For this review, take the finished solid that the model builds, in its own axes (mm). Face numbers are marked on the shaded views. A direction names the side the tool comes from. Give positions to 0.01 mm unless a question says otherwise; leave off trailing zeros. Order: outer loops, then holes, each group sorted by start corner. A loop starts at its lowest first (then second) coordinate and runs counter-clockwise, first axis right, second up.
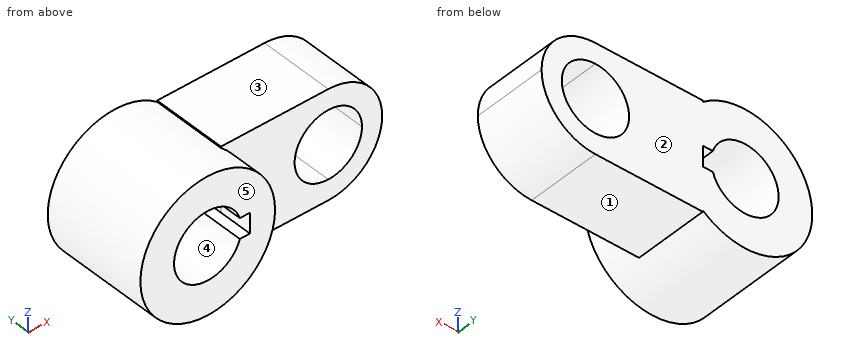
from build123d import *

# Parameters (mm, degrees)
F1_DEPTH = 34.925
F2_R     = 31.75
F3_DEPTH = 50.8


with BuildPart() as f1:
    # F0 (on Front) → F1 (new body)
    with BuildSketch(Plane.XZ):
        with BuildLine():
            Line((38.1, 25.4), (-9.5485188067, 25.4))
            Line((-9.5485188067, 25.4), (-12.5222, 25.4))
            Line((-12.5222, 25.4), (-12.5222, -25.4))
            Line((-12.5222, -25.4), (-9.5485188067, -25.4))
            Line((-9.5485188067, -25.4), (38.1, -25.4))
            ThreePointArc((38.1, -25.4), (12.7, 0), (38.1, 25.4))
        make_face()
        with BuildLine():
            ThreePointArc((63.5, 0), (56.0605122421, 17.9605122421), (38.1, 25.4))
            Line((38.1, 25.4), (38.1, 15.875))
            ThreePointArc((38.1, 15.875), (49.3253201513, 11.2253201513), (53.975, 0))
            ThreePointArc((53.975, 0), (49.3253201513, -11.2253201513), (38.1, -15.875))
            Line((38.1, -15.875), (38.1, -25.4))
            ThreePointArc((38.1, -25.4), (56.0605122421, -17.9605122421), (63.5, 0))
        make_face()
        with BuildLine():
            Line((38.1, 15.875), (38.1, 25.4))
            ThreePointArc((38.1, 25.4), (12.7, 0), (38.1, -25.4))
            Line((38.1, -25.4), (38.1, -15.875))
            ThreePointArc((38.1, -15.875), (22.225, 0), (38.1, 15.875))
        make_face()
    extrude(amount=F1_DEPTH)

    # F2 (on Front) → F3 (join)
    with BuildSketch(Plane.XZ):
        with Locations((-32.41843798, 0)):
            Circle(F2_R)
        with BuildLine():
            ThreePointArc((-17.2746531575, -4.7625), (-48.29343798, 0), (-17.2746531575, 4.7625))
            Line((-17.2746531575, 4.7625), (-12.5121531575, 4.7625))
            Line((-12.5121531575, 4.7625), (-12.5121531575, -4.7625))
            Line((-12.5121531575, -4.7625), (-17.2746531575, -4.7625))
        make_face(mode=Mode.SUBTRACT)
    extrude(amount=F3_DEPTH)


solid = f1.part
1) Clearance check with flat-ended pins moving along their axes: pin 1 (12 mm diameter, centred on y = -36.5, z = 17, fed in from -X); pin 2 (4 mm diameter, centred on x = -15.5, y = -30.5, fed in from -Z); pin 3 (1.5 mm diameter, centred on x = 11, z = -21, fed in from -Y) (3 decimals). State where each tip first meets the part, or that it passes through.
Answer sheet:
pin 1: stops at x = -62.2
pin 2: stops at z = -28.03
pin 3: stops at y = -34.925
2) We need section C-C on y = -20.5. Count the separate pieces of the cut face and the enclosed holes in it, then the cut area to 3 significant figures.
Answer sheet:
separate pieces: 1
enclosed holes: 2
area: 4,720 mm2
3) Tool access review of the marked faces 1, 2 and 3: name each direction out of +Z, -Z, +X, -X, +Y, -Y from which nothing blocks a thin tool from reaching the whole face with its end or side.
Answer sheet:
face 1: -Z, +X, +Y, -Y
face 2: +Z, -Z, +X, -X, +Y
face 3: +Z, +X, +Y, -Y
4) To check wall thickness, follow line 1 (X direction, y = -15, z = -12.5); line 2 (X direction, y = -19, z = 4); line 3 (Z direction, x = -33, y = -40). State the ranges of each line that lie inside material, in increasing order.
Answer sheet:
line 1: x = -61.6 to -42.2, -22.63 to 28.31, 47.89 to 60.21
line 2: x = -63.92 to -47.78, -12.52 to 22.74, 53.46 to 63.18
line 3: z = -31.74 to -15.86, 15.86 to 31.74
5) We need section A-A on x = -41. Give the boundary of the cut face in (y, z).
Answer sheet:
outline: (-50.8, -30.57) - (0, -30.57) - (0, -13.36) - (-50.8, -13.36) - close; (-50.8, 13.36) - (0, 13.36) - (0, 30.57) - (-50.8, 30.57) - close
6) We need section B-B on z = 12. Give the boundary of the cut face in (x, y) (1 decimal), then the cut area to 3 significant figures.
Answer sheet:
outline: (-61.8, -50.8) - (-42.8, -50.8) - (-42.8, 0) - (-61.8, 0) - close; (-22, -50.8) - (-3, -50.8) - (-3, -34.9) - (27.7, -34.9) - (27.7, 0) - (-22, 0) - close; (48.5, -34.9) - (60.5, -34.9) - (60.5, 0) - (48.5, 0) - close
area: 3,420 mm2
7) Draft analysis for pull direction X (two halves, no side actions). For the marked faces 4 and 5, state which applies: +X half, -X half, draft (parallel to the pull), parting line (faces both ways), or undercut.
Answer sheet:
face 4: undercut
face 5: draft
